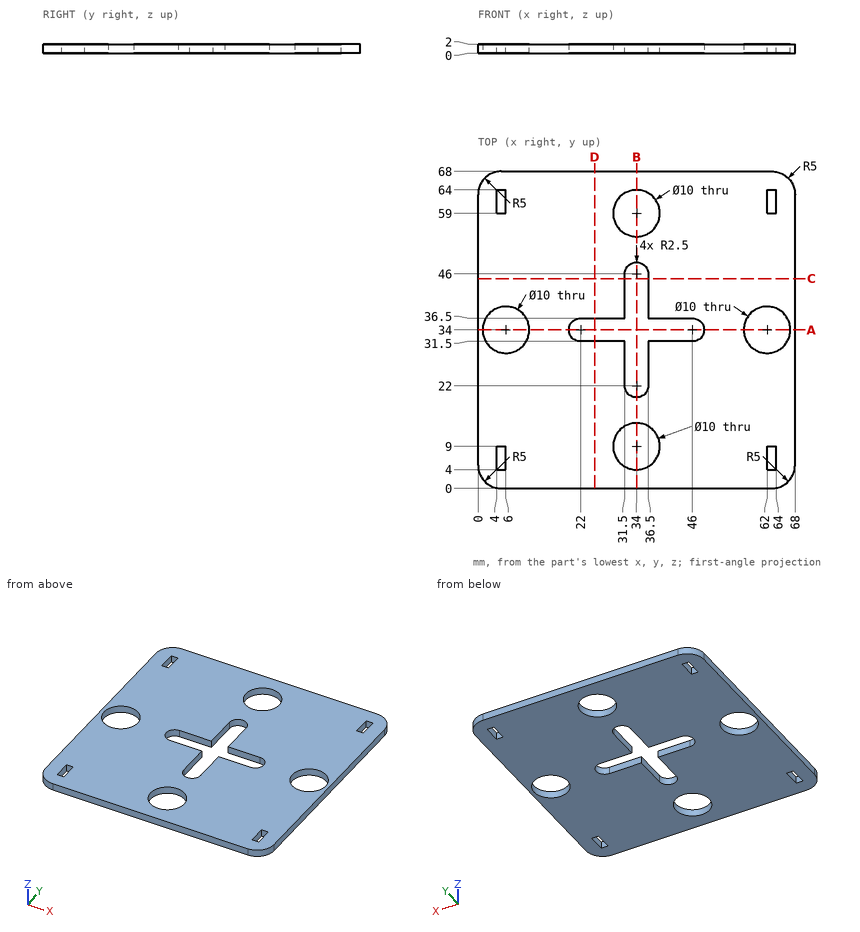
Print and shaded views of the part. All mm, measured from the part's lowest x, y and z. Give positions to 0.01 mm unless a question says otherwise; leave off trailing zeros. Loops run counter-clockwise (first coordinate to the right, second up) from the corner with the lowest first, then second, coordinate; pieces in that order, holes last.
1) Saw through at A-A (y = 34). Write the cut outline in (x, z), plus the area to 3 significant figures.
2) Wall check: line 1 (Y direction, x = 34, z = 1.2); line 2 (X direction, y = 42, z = 1); line 3 (Y direction, x = 62.5, z = 1.7). Give the ranges that are in metal, low to high.
3) Saw through at C-C (y = 45). Write the cut outline in (x, z).
4) Saw through at B-B (x = 34). Write the cut outline in (y, z), plus the area to 3 significant figures.
Answer block:
1. outline: (0, 0) - (1, 0) - (1, 2) - (0, 2) - close; (11, 0) - (19.5, 0) - (19.5, 2) - (11, 2) - close; (48.5, 0) - (57, 0) - (57, 2) - (48.5, 2) - close; (67, 0) - (68, 0) - (68, 2) - (67, 2) - close
1. area: 38.0 mm2
2. line 1: y = 0 to 4, 14 to 19.5, 48.5 to 54, 64 to 68
2. line 2: x = 0 to 31.5, 36.5 to 68
2. line 3: y = 0 to 4, 9 to 29.03, 38.97 to 59, 64 to 68
3. outline: (0, 0) - (31.5, 0) - (31.5, 2) - (0, 2) - close; (36.5, 0) - (68, 0) - (68, 2) - (36.5, 2) - close
4. outline: (0, 0) - (4, 0) - (4, 2) - (0, 2) - close; (14, 0) - (19.5, 0) - (19.5, 2) - (14, 2) - close; (48.5, 0) - (54, 0) - (54, 2) - (48.5, 2) - close; (64, 0) - (68, 0) - (68, 2) - (64, 2) - close
4. area: 38.0 mm2
